```python
from build123d import *

# Parameters (mm, degrees)
SKETCH1_W           = 19.05
SKETCH1_H           = 57.15
BOSS_EXTRUDE1_DEPTH = 50.8
SKETCH1_4_R         = 6.35
CUT_EXTRUDE1_DEPTH  = 60.05841388
SKETCH1_5_R         = 2.54
BOSS_EXTRUDE2_DEPTH = 50.8
SKETCH1_6_R         = 6.35
CUT_EXTRUDE2_DEPTH  = 60.05841388
SKETCH1_7_R         = 2.54
BOSS_EXTRUDE3_DEPTH = 50.8
SKETCH11_W          = 19.05
SKETCH11_H          = 50.8
CUT_EXTRUDE12_DEPTH = 2.54
SKETCH12_W          = 19.05
SKETCH12_H          = 50.8
BOSS_EXTRUDE4_DEPTH = 12.7
SKETCH13_R          = 3.81
CUT_EXTRUDE15_DEPTH = 69.170141008
SKETCH13_6_W        = 2.54
SKETCH13_6_H        = 6.35
CUT_EXTRUDE16_DEPTH = 69.170141008
SKETCH13_7_R        = 1.5875
CUT_EXTRUDE17_DEPTH = 69.170141008


with BuildPart() as part:
    # Sketch1 → Boss-Extrude1 (new body)
    with BuildSketch(Plane.XY):
        Rectangle(SKETCH1_W, SKETCH1_H)
    extrude(amount=BOSS_EXTRUDE1_DEPTH)

    # Sketch1<4> → Cut-Extrude1 (cut, through all)
    with BuildSketch(Plane.XY):
        with Locations((0, -15.875)):
            Circle(SKETCH1_4_R)
    extrude(amount=CUT_EXTRUDE1_DEPTH, mode=Mode.SUBTRACT)

    # Sketch1<5> → Boss-Extrude2 (add, through all)
    with BuildSketch(Plane.XY):
        with Locations((0, -9.525)):
            Circle(SKETCH1_5_R)
        with Locations((5.499261314, -19.05)):
            Circle(SKETCH1_5_R)
        with Locations((-5.499261314, -19.05)):
            Circle(SKETCH1_5_R)
    extrude(amount=BOSS_EXTRUDE2_DEPTH)

    # Sketch1<6> → Cut-Extrude2 (cut, through all)
    with BuildSketch(Plane.XY):
        with Locations((0, 15.875)):
            Circle(SKETCH1_6_R)
    extrude(amount=CUT_EXTRUDE2_DEPTH, mode=Mode.SUBTRACT)

    # Sketch1<7> → Boss-Extrude3 (add, through all)
    with BuildSketch(Plane.XY):
        with Locations((0, 22.225)):
            Circle(SKETCH1_7_R)
        with Locations((5.499261314, 12.7)):
            Circle(SKETCH1_7_R)
        with Locations((-5.499261314, 12.7)):
            Circle(SKETCH1_7_R)
    extrude(amount=BOSS_EXTRUDE3_DEPTH)

    # Sketch11 → Cut-Extrude12 (cut)
    with BuildSketch(Plane(origin=(0, 28.575, 0), x_dir=(1, 0, 0), z_dir=(0, 1, 0))):
        with Locations((0, -25.4)):
            Rectangle(SKETCH11_W, SKETCH11_H)
    extrude(amount=-CUT_EXTRUDE12_DEPTH, mode=Mode.SUBTRACT)

    # Sketch12 → Boss-Extrude4 (add)
    with BuildSketch(Plane.XZ.offset(28.575)):
        with Locations((0, 25.4)):
            Rectangle(SKETCH12_W, SKETCH12_H)
    extrude(amount=BOSS_EXTRUDE4_DEPTH)

    # Sketch13 → Cut-Extrude15 (cut, through all)
    with BuildSketch(Plane(origin=(9.525, 0, 0), x_dir=(0, 0, -1), z_dir=(1, 0, 0))):
        with Locations(Location((-43.18, -31.75, 0), (0, 0, 90))):
            Circle(SKETCH13_R)
        with Locations(Location((-7.62, -31.75, 0), (0, 0, 90))):
            Circle(SKETCH13_R)
    extrude(amount=-CUT_EXTRUDE15_DEPTH, mode=Mode.SUBTRACT)

    # Sketch13<6> → Cut-Extrude16 (cut, through all)
    with BuildSketch(Plane(origin=(9.525, 0, 0), x_dir=(0, 0, -1), z_dir=(1, 0, 0))):
        with Locations((-25.4, -31.75)):
            Rectangle(SKETCH13_6_W, SKETCH13_6_H)
    extrude(amount=-CUT_EXTRUDE16_DEPTH, mode=Mode.SUBTRACT)

    # Sketch13<7> → Cut-Extrude17 (cut, through all)
    with BuildSketch(Plane(origin=(9.525, 0, 0), x_dir=(0, 0, -1), z_dir=(1, 0, 0))):
        with Locations(Location((-19.05, -28.575, 0), (0, 0, 90))):
            Circle(SKETCH13_7_R)
        with Locations(Location((-19.05, -34.925, 0), (0, 0, 90))):
            Circle(SKETCH13_7_R)
    extrude(amount=-CUT_EXTRUDE17_DEPTH, mode=Mode.SUBTRACT)


solid = part.part
```
Input: part model. Units: mm. Frame: model coordinates. A direction names the side the tool comes from. Coordinates: 2 decimals unless noted, no trailing zeros. Write each loop counter-clockwise with the first axis right and the second up, starting at its lowest first coordinate (ties: lowest second). Pieces come first, ordered by that corner, then holes. Notation, with made-up numbers: M -22.75,15 L -9.75,15 A10 cw -9.75,19 Z; hole C 83,31.5 d2. An arc over 180 degrees is marked long. Use one line per item in the form item = value.
Q1. Section B-B (z = 43.18). Return loops of the section in (x, y) (3 decimals), plus the area to 3 significant figures.
Answer below:
outline = M -9.525,-41.275 L 9.525,-41.275 L 9.525,-35.56 L -9.525,-35.56 Z; M -9.525,-27.94 L 9.525,-27.94 L 9.525,26.035 L -9.525,26.035 Z; hole M -6.304,-16.641 A2.54 cw -3.815,-20.951 A6.35 ccw 3.815,-20.951 A2.54 cw 6.304,-16.641 A6.35 ccw 2.489,-10.033 A2.54 cw -2.489,-10.033 A6.35 ccw Z; hole M -6.304,15.109 A2.54 cw -3.815,10.799 A6.35 ccw 3.815,10.799 A2.54 cw 6.304,15.109 A6.35 ccw 2.489,21.717 A2.54 cw -2.489,21.717 A6.35 ccw Z
area = 939 mm²
Q2. Draft query along Y for faces 1 (the face through (0, -7, 0)), 2 (the face through (-3.276, -17.822, 25.044)), 3 (the face through (0, -41.275, 26)), 4 (the face through (0, 26.035, 25)). Return one class per face: released by +Y, released by -Y, zero draft, split by the parting line, or undercut.
Answer below:
face_1 = zero draft
face_2 = undercut
face_3 = released by -Y
face_4 = released by +Y
Q3. Set-up query: faces 5 (the face through (0, -34.925, 25)), 6 (the face through (0, -7, 50.8)). Return all of +Z, -Z, +X, -X, +Y, -Y with unobstructed straight access to the full face (end or side cutting, diameter ignored); none if empty.
Answer below:
face_5 = +X, -X
face_6 = +Z, +X, -X, +Y, -Y
Q4. Section A-A (z = 19.05). Count the separate pieces of the cut face and the enclosed holes in it, plus the area to 3 significant figures.
Answer below:
separate_pieces = 3
enclosed_holes = 2
area = 964 mm²
Q5. Section D-D (y = -31.75). Return loops of the section in (x, z) (3 decimals).
Answer below:
outline = M -9.525,0 L 9.525,0 L 9.525,3.81 L -9.525,3.81 Z; M -9.525,11.43 L 9.525,11.43 L 9.525,24.13 L -9.525,24.13 Z; M -9.525,26.67 L 9.525,26.67 L 9.525,39.37 L -9.525,39.37 Z; M -9.525,46.99 L 9.525,46.99 L 9.525,50.8 L -9.525,50.8 Z
Q6. Material intervals for probe 1 along Z at (x, y) = (5.25, -31.75); probe 2 along Y at (x, z) = (7.25, 19) (3 decimals); probe 3 along Y at (x, z) = (-3.5, 47.5) (3 decimals), sorted ascending. Write a range as from..to.
Answer below:
probe_1 = 0..3.81, 11.43..24.13, 26.67..39.37, 46.99..50.8
probe_2 = -41.275..-36.512, -33.338..-30.162, -26.988..26.035
probe_3 = -41.275..-21.173, -20.617..-17.483, -10.577..10.577, 11.133..14.267, 21.173..26.035
